Source: CAD feature listing. Evaluate the final solid. Frame: model axes, mm. Face numbers are marked on the shaded views. A direction names the side the tool comes from. Round coordinates to 2 decimals unless told otherwise and drop trailing zeros. Loops run counter-clockwise (first coordinate to the right, second up) from the corner with the lowest first, then second, coordinate; pieces in that order, holes last.
Item 1: Section query C-C on y = 6.58. Return loops of the section in (x, z).
Item 2: First-contact query: P1, Ø7, axis at x = -0.5, y = -15, coming from the +Z side; P2, Ø8, axis at x = 31.5, y = -3.5, coming from the -Z side; P3, Ø2.5, axis at x = 48.02, y = -4.9, coming from the -Z side; P4, Ø3, axis at x = 19.5, z = 30.5, coming from the -Y side. Flat tips, straight axial feed; report the tip coordinate or a pass-through.
Item 3: Section query D-D on z = 28. Return loops of the section in (x, y).
Item 4: Access query for the marked faces 4, 5 and 6. Directions: +Z, -Z, +X, -X, +Y, -Y. A direction counts if a zero-diameter tool reaches every point of the face in a straight line with its end or side. Return the directions, or none.
Item 5: Section query A-A on y = -2. Return loops of the section in (x, z), then the cut area to 3 significant figures.
Item 6: Ray query, L1, parallel to X at y = -4, z = 33; L2, parallel to Y at x = 42.5, z = 32.5; L3, parallel to Y at x = 44.5, z = 34.5. Return the intervals inside material, ascending.
Item 7: Section query B-B on y = -16.5. Return loops of the section in (x, z).
Item 8: Pull-direction query (Z, two-part tool) for the marked faces 1, 2 and 3; classes: released by +Z, released by -Z, zero draft, split by the parting line, or undercut.
```python
from build123d import *

# Parameters (mm, degrees)
SKETCH1_W                = 53
SKETCH1_H                = 30.745586227
BOSS_EXTRUDE1_DEPTH      = 3
SKETCH2_W                = 6.5
SKETCH2_H                = 3
BOSS_EXTRUDE2_DEPTH      = 20
SKETCH3_R                = 2.15
CUT_EXTRUDE1_DEPTH       = 3
SKETCH6_W                = 17
SKETCH6_H                = 7.58
BOSS_EXTRUDE3_DEPTH      = 3
SKETCH7_R                = 1.5
CUT_EXTRUDE2_DEPTH       = 7.5
SKETCH8_W                = 6
SKETCH8_H                = 14
CUT_EXTRUDE3_DEPTH       = 0.5
BOSS_EXTRUDE4_DEPTH      = 2
BOSS_EXTRUDE4_DEPTH_BACK = 2
BOSS_EXTRUDE5_DEPTH      = 3


with BuildPart() as part:
    # Sketch1 → Boss-Extrude1 (new body)
    with BuildSketch(Plane(origin=(0, 0, 0), x_dir=(1, 0, 0), z_dir=(0, 1, 0))):
        with Locations((24.118089155, -22.118099476)):
            Rectangle(SKETCH1_W, SKETCH1_H)
    extrude(amount=BOSS_EXTRUDE1_DEPTH)

    # Sketch2 → Boss-Extrude2 (add)
    with BuildSketch(Plane.XZ):
        with Locations((47.368089155, 33.49089259)):
            Rectangle(SKETCH2_W, SKETCH2_H)
        with Locations((0.868089155, 33.49089259)):
            Rectangle(SKETCH2_W, SKETCH2_H)
    extrude(amount=BOSS_EXTRUDE2_DEPTH)

    # Sketch3 → Cut-Extrude1 (cut)
    with BuildSketch(Plane.XY.offset(34.99089259)):
        with Locations((48.018089155, -15.1)):
            Circle(SKETCH3_R)
        with Locations((48.018089155, -4.9)):
            Circle(SKETCH3_R)
        with Locations((0.218089155, -15.1)):
            Circle(SKETCH3_R)
        with Locations((0.218089155, -4.9)):
            Circle(SKETCH3_R)
    extrude(amount=-CUT_EXTRUDE1_DEPTH, mode=Mode.SUBTRACT)

    # Sketch6 → Boss-Extrude3 (add)
    with BuildSketch(Plane.XY.offset(37.49089259)):
        with Locations((6.118089155, 6.79)):
            Rectangle(SKETCH6_W, SKETCH6_H)
    extrude(amount=-BOSS_EXTRUDE3_DEPTH)

    # Sketch7 → Cut-Extrude2 (cut)
    with BuildSketch(Plane.XY.offset(37.49089259)):
        with Locations((0.118089155, 6.58)):
            Circle(SKETCH7_R)
        with Locations((11.618089155, 6.58)):
            Circle(SKETCH7_R)
    extrude(amount=-CUT_EXTRUDE2_DEPTH, mode=Mode.SUBTRACT)

    # Sketch8 → Cut-Extrude3 (cut)
    with BuildSketch(Plane(origin=(0, 3, 0), x_dir=(1, 0, 0), z_dir=(0, 1, 0))):
        with Locations((11.618089155, -27.49089259)):
            Rectangle(SKETCH8_W, SKETCH8_H)
        with Locations((0.618089155, -27.49089259)):
            Rectangle(SKETCH8_W, SKETCH8_H)
    extrude(amount=-CUT_EXTRUDE3_DEPTH, mode=Mode.SUBTRACT)

    # Sketch13 → Boss-Extrude4 (add, two sides: drawn at the far end of the back side and taken through both)
    with BuildSketch(Plane.ZY.offset(-6.118089155).offset(-BOSS_EXTRUDE4_DEPTH_BACK)):
        Polygon((34.49089259, 10.57033397), (34.49089259, 3), (20.468920989, 3), align=None)
    extrude(amount=BOSS_EXTRUDE4_DEPTH + BOSS_EXTRUDE4_DEPTH_BACK)

    # Sketch14 → Boss-Extrude5 (add)
    with BuildSketch(Plane.XY.offset(37.49089259)):
        Polygon((14.618089155, 3), (14.618089155, 10.58), (21.91210821, 3), align=None)
    extrude(amount=-BOSS_EXTRUDE5_DEPTH)


solid = part.part
```
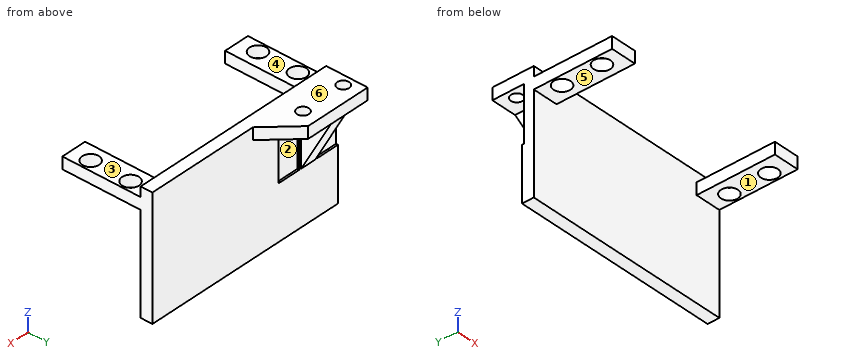
Data:
1. outline: (-2.38, 34.49) - (-1.38, 34.49) - (-1.38, 37.49) - (-2.38, 37.49) - close; (1.62, 34.49) - (4.12, 34.49) - (4.12, 27.1) - (8.12, 27.1) - (8.12, 34.49) - (10.12, 34.49) - (10.12, 37.49) - (1.62, 37.49) - close; (13.12, 34.49) - (18.47, 34.49) - (18.47, 37.49) - (13.12, 37.49) - close
2. P1: stops at z = 34.99
2. P2: stops at z = 6.75
2. P3: passes through
2. P4: stops at y = 0
3. outline: (-2.38, 0) - (50.62, 0) - (50.62, 3) - (14.62, 3) - (14.62, 2.5) - (8.62, 2.5) - (8.62, 3) - (8.12, 3) - (8.12, 7.07) - (4.12, 7.07) - (4.12, 3) - (3.62, 3) - (3.62, 2.5) - (-2.38, 2.5) - close
4. face 4: +Z, +X, -X, -Y
4. face 5: -Z, +X, -X, -Y
4. face 6: +Z, +X, -X, +Y, -Y
5. outline: (-2.38, 31.99) - (4.12, 31.99) - (4.12, 34.99) - (-2.38, 34.99) - close; (44.12, 31.99) - (50.62, 31.99) - (50.62, 34.99) - (44.12, 34.99) - close
5. area: 39.0 mm2
6. L1: x = -2.38 to -1.73, 2.17 to 4.12, 44.12 to 46.07, 49.97 to 50.62
6. L2: y = 0 to 3
6. L3: y = -20 to 3
7. outline: (-2.38, 31.99) - (-1.41, 31.99) - (-1.41, 34.99) - (-2.38, 34.99) - close; (1.85, 31.99) - (4.12, 31.99) - (4.12, 34.99) - (1.85, 34.99) - close; (44.12, 31.99) - (46.39, 31.99) - (46.39, 34.99) - (44.12, 34.99) - close; (49.65, 31.99) - (50.62, 31.99) - (50.62, 34.99) - (49.65, 34.99) - close
8. face 1: released by -Z
8. face 2: undercut
8. face 3: released by +Z
